Source: CAD feature listing. Evaluate the final solid. Frame: model axes, mm. A direction names the side the tool comes from. Round coordinates to 2 decimals unless told otherwise and drop trailing zeros. Order: outer loops, then holes, each group sorted by start corner. A loop starts at its lowest first (then second) coordinate and runs counter-clockwise, first axis right, second up. Notation, with made-up numbers: (3.5, 13) -> (58.5, 13) arc R8 ccw to (58.5, 26) -> close; hole circle Ø4 at (6, 2). An arc over 180 degrees is marked (long way). Answer as CSV lines item,"result".
from build123d import *

# Parameters (mm, degrees)
SKETCH1_W           = 40
SKETCH1_H           = 20
BOSS_EXTRUDE1_DEPTH = 40
SKETCH2_R           = 1.340799443
BOSS_EXTRUDE2_DEPTH = 2.5
SKETCH3_W           = 40
SKETCH3_H           = 10
CUT_EXTRUDE1_DEPTH  = 20
SKETCH5_W           = 10
SKETCH5_H           = 30
CUT_EXTRUDE4_DEPTH  = 20


with BuildPart() as part:
    # Sketch1 → Boss-Extrude1 (new body)
    with BuildSketch(Plane.XY):
        with Locations((-12.31884058, 10.869565217)):
            Rectangle(SKETCH1_W, SKETCH1_H)
    extrude(amount=BOSS_EXTRUDE1_DEPTH)

    # Sketch2 → Boss-Extrude2 (add)
    with BuildSketch(Plane.XY.offset(40)):
        with Locations((-28.31884058, 10.869565217)):
            Circle(SKETCH2_R)
    extrude(amount=BOSS_EXTRUDE2_DEPTH)

    # Sketch3 → Cut-Extrude1 (cut)
    with BuildSketch(Plane.XZ.offset(-0.869565217)):
        with Locations((-12.31884058, 5)):
            Rectangle(SKETCH3_W, SKETCH3_H)
    extrude(amount=-CUT_EXTRUDE1_DEPTH, mode=Mode.SUBTRACT)

    # Sketch5 → Cut-Extrude4 (cut)
    with BuildSketch(Plane.XZ.offset(-0.869565217)):
        with Locations((2.68115942, 25)):
            Rectangle(SKETCH5_W, SKETCH5_H)
    extrude(amount=-CUT_EXTRUDE4_DEPTH, mode=Mode.SUBTRACT)


solid = part.part
1. Pin query (flat end, axial travel): pin 1 (1 mm diameter, centred on x = -22.5, y = 17.5, fed in from +Z). Return the tip coordinate at first contact, or that it passes through.
Results below:
pin 1,"z = 40"
2. Section query D-D on y = 18.25. Return loops of the section in (x, z).
Results below:
outline,"(-32.32, 10) -> (-2.32, 10) -> (-2.32, 40) -> (-32.32, 40) -> close"
3. Reachability of faces 1 (the cylindrical face through (-29.66, 10.93, 41.23)), 2 (the flat face through (-18, 20.87, 25)) from +Z, -Z, +X, -X, +Y, -Y: full face, straight path, thin tool, end or side. Return the list, or none.
Results below:
face 1,"+Z"
face 2,"+Z, -Z, +X, -X, +Y"
4. Section query A-A on x = -27.5. Return loops of the section in (y, z), and give its area (3 significant figures).
Results below:
outline,"(0.87, 10) -> (20.87, 10) -> (20.87, 40) -> (11.93, 40) -> (11.93, 42.5) -> (9.81, 42.5) -> (9.81, 40) -> (0.87, 40) -> close"
area,"605 mm2"
5. Line query: L1, parallel to Z at x = -20, y = 14. Output: solid intervals per line, ascending. Write a range as [from, to].
Results below:
L1,"[10, 40]"
6. Section query C-C on x = -14.5. Return loops of the section in (y, z), and give its area (3 significant figures).
Results below:
outline,"(0.87, 10) -> (20.87, 10) -> (20.87, 40) -> (0.87, 40) -> close"
area,"600 mm2"
7. Section query B-B on y = 10. Return loops of the section in (x, z), and give its area (3 significant figures).
Results below:
outline,"(-32.32, 10) -> (-2.32, 10) -> (-2.32, 40) -> (-27.3, 40) -> (-27.3, 42.5) -> (-29.34, 42.5) -> (-29.34, 40) -> (-32.32, 40) -> close"
area,"905 mm2"
